Autodesk Inventor part; units mm, degrees
ref_plane "YZ Plane" through (0, 0, 0) normal (1, 0, 0) x (0, 1, 0)
ref_plane "XZ Plane" through (0, 0, 0) normal (0, 1, 0) x (-1, 0, 0)
ref_plane "XY Plane" through (0, 0, 0) normal (0, 0, 1) x (1, 0, 0)
sketch "Szkic1" plane through (0, 0, 0) normal (0, 1, 0) x (-1, 0, 0)
  line L0 (30, -20) -> (-30, -20)
  line L1 (-30, -20) -> (-30, 20)
  line L2 (-30, 20) -> (30, 20)
  line L3 (30, 20) -> (30, -20)
  line L4 (30, -20) -> (-30, 20) construction
  line L5 (-30, -20) -> (30, 20) construction
  point P0 (0, 0)
  dimension "d0" = 60
  dimension "d1" = 40
extrude "Wyciągnięcie proste1" add sketch "Szkic1" along normal blind 3
sketch "Szkic6" plane through (0, 3, 0) normal (0, 1, 0) x (1, 0, 0)
  line L0 (17.3578, -5.5734) -> (12.5578, -5.5734)
  line L1 (12.5578, -5.5734) -> (12.5578, 12.7266)
  line L2 (12.5578, 12.7266) -> (-10.1422, 12.7266)
  line L3 (-10.1422, -5.5734) -> (-10.1422, 12.7266)
  line L4 (-10.1422, -5.5734) -> (-14.9422, -5.5734)
  line L5 (-14.9422, -5.5734) -> (-14.9422, -8.2734)
  line L6 (-10.1422, -8.2734) -> (-14.9422, -8.2734)
  line L7 (-10.1422, -8.2734) -> (-10.1422, -10.0734)
  line L8 (-10.1422, -10.0734) -> (12.5578, -10.0734) construction
  line L9 (12.5578, -8.2734) -> (12.5578, -10.0734)
  line L10 (17.3578, -8.2734) -> (12.5578, -8.2734)
  line L11 (17.3578, -5.5734) -> (17.3578, -8.2734)
  line L12 (-8.8922, -2.4734) -> (11.3078, -2.4734)
  line L13 (-8.8922, 7.7266) -> (-8.8922, -2.4734)
  line L14 (11.3078, 7.7266) -> (-8.8922, 7.7266)
  line L15 (11.3078, -2.4734) -> (11.3078, 7.7266)
  line L16 (-30, -20) -> (30, -20)
  line L17 (30, -20) -> (30, 20)
  line L18 (30, -20) -> (30, 20)
  line L19 (-30, 20) -> (-30, -20)
  line L20 (-30, -20) -> (-14.5223, -20)
  line L21 (23.4752, -20) -> (30, -20)
  line L22 (-10.6422, 13.2266) -> (13.0578, 13.2266)
  line L23 (13.4777, 6.2814) -> (13.4777, -4.6535)
  line L24 (13.4777, -4.6535) -> (18.2777, -4.6535)
  line L25 (18.2777, -4.6535) -> (18.2777, -9.1933)
  line L26 (18.2777, -9.1933) -> (13.4777, -9.1933)
  line L27 (13.4777, -9.1933) -> (13.4777, -10.5734)
  line L28 (-10.6422, -10.5734) -> (-10.6422, -8.7734)
  line L29 (-10.6422, -8.7734) -> (-15.4422, -8.7734)
  line L30 (-15.4422, -8.7734) -> (-15.4422, -5.0734)
  line L31 (-15.4422, -5.0734) -> (-10.6422, -5.0734)
  line L32 (-10.6422, -5.0734) -> (-10.6422, 13.2266)
  line L33 (13.4777, -10.5734) -> (23.4752, -20)
  line L34 (-10.6422, -10.5734) -> (-14.5223, -20)
  line L35 (13.4777, 6.2814) -> (16.9504, 6.2814)
  line L36 (16.9504, 6.2814) -> (16.9504, 20)
  line L37 (13.0578, 13.2266) -> (13.0578, 20)
  line L38 (30, 20) -> (16.9504, 20)
  line L39 (13.0578, 20) -> (-30, 20)
  point P0 (0, 0)
  dimension "d4" = 0.5
extrude "Wyciągnięcie proste2" add sketch "Szkic6" along normal blind 13 contours L19 L39 L37 L22 L32 L31 L30 L29 L28 L34 L16 | L33 L27 L26 L25 L24 L23 L35 L36 L38 L17 L16
sketch "Szkic7" plane through (0, 3, 0) normal (0, 1, 0) x (1, 0, 0)
  line L0 (13.0578, 20) -> (13.0578, 13.2266)
  line L1 (13.0578, 13.2266) -> (-10.6422, 13.2266)
  line L2 (-10.6422, 13.2266) -> (-10.6422, -5.0734)
  line L3 (-10.6422, -5.0734) -> (-15.4422, -5.0734)
  line L4 (-15.4422, -5.0734) -> (-15.4422, -8.7734)
  line L5 (-15.4422, -8.7734) -> (-10.6422, -8.7734)
  line L6 (-10.6422, -8.7734) -> (-10.6422, -10.5734)
  line L7 (-10.6422, -10.5734) -> (-14.5223, -20)
  line L8 (-14.5223, -20) -> (23.4752, -20)
  line L9 (23.4752, -20) -> (13.4777, -10.5734)
  line L10 (13.4777, -10.5734) -> (13.4777, -9.1933)
  line L11 (13.4777, -9.1933) -> (18.2777, -9.1933)
  line L12 (18.2777, -9.1933) -> (18.2777, -4.6535)
  line L13 (18.2777, -4.6535) -> (13.4777, -4.6535)
  line L14 (13.4777, -4.6535) -> (13.4777, 6.2814)
  line L15 (13.4777, 6.2814) -> (16.9504, 6.2814)
  line L16 (16.9504, 6.2814) -> (16.9504, 20)
  line L17 (16.9504, 20) -> (13.0578, 20)
  line L18 (1.3504, -15.7734) -> (12.6578, -15.7734)
  line L19 (-12.7826, -15.7734) -> (18.9926, -15.7734)
  point P0 (0, 0)
  point P1 (12.6578, -15.7734)
  point P2 (1.3504, -15.7734)
extrude "Wyciągnięcie proste3" cut sketch "Szkic7" against normal blind 13 contours L19 L18 L9 L8 L7
sketch "Szkic8" plane through (0, 16, 0) normal (0, 1, 0) x (1, 0, 0)
  line L0 (-30, 20) -> (-30, -20)
  line L1 (-30, -20) -> (-14.5223, -20)
  line L2 (30, 20) -> (-30, 20)
  line L3 (-30, 0) -> (30, 0) construction
  line L4 (0, 20) -> (0, -29.6332) construction
  point P0 (0, 0)
  point P1 (-25, -15)
  point P2 (-25, 15)
  point P3 (25, 15)
  point P4 (25, -15)
  dimension "d9" = 5
  dimension "d10" = 5
hole "Otwór1" at (-25, 16, 15) at (-25, 16, -15) at (25, 16, -15) at (25, 16, 15) direction (0, -1, 0) diameter 4.134 depth 5 tip angle 118
sketch "Szkic9" plane through (0, 0, 0) normal (0, -1, 0) x (1, 0, 0)
  line L0 (30, 20) -> (30, -20)
  line L1 (30, -20) -> (-30, -20)
  line L2 (-30, -20) -> (-30, -17)
  line L3 (-30, -17) -> (30, -17)
  line L4 (30, -17) -> (30, -20)
  line L5 (18.9926, 15.7734) -> (-12.7826, 15.7734)
  line L6 (30, 20) -> (23.4752, 20)
  line L7 (23.4752, 17) -> (30, 17)
  line L8 (30, 17) -> (30, 20)
  line L9 (23.4752, 20) -> (18.9926, 15.7734)
  line L10 (23.4752, 20) -> (23.4752, 17)
  line L11 (-30, 20) -> (-14.5223, 20)
  line L12 (-30, 20) -> (-14.5223, 20)
  line L13 (-14.5223, 17) -> (-30, 17)
  line L14 (-30, 17) -> (-30, 20)
  line L15 (-14.5223, 20) -> (-10.6422, 10.5734)
  line L16 (-14.5223, 20) -> (-14.5223, 17)
  point P0 (0, 0)
  dimension "d18" = 60
  dimension "d19" = 3
  dimension "d31" = 3
  dimension "d32" = 3
extrude "Wyciągnięcie proste4" add sketch "Szkic9" along normal blind 3
sketch "Szkic10" plane through (0, 16, 0) normal (0, 1, 0) x (1, 0, 0)
  line L0 (-30, 20) -> (-30, -20)
  line L1 (30, -20) -> (30, 20)
  point P0 (0, 0)
  point P1 (-20, 0)
  point P2 (20, 0)
  dimension "d22" = 10
  dimension "d23" = 10
hole "Otwór2" at (-20, 16, 0) at (20, 16, 0) direction (0, -1, 0) diameter 4.134 end through all
properties part number "Podstawa"
The model under review builds one solid part; all positions refer to its coordinate system, in mm. A direction names the side the tool comes from. Round coordinates to 2 decimals unless told otherwise and drop trailing zeros. Loops run counter-clockwise (first coordinate to the right, second up) from the corner with the lowest first, then second, coordinate; pieces in that order, holes last.
Item 1: Clearance check with flat-ended pins moving along their axes: pin 1 Ø12 at (x, z) = (9.5, -4.5) entering from +Y; pin 2 Ø1.4 at (x, y) = (-12, 12) entering from +Z; pin 3 Ø5 at (x, y) = (10.5, 4) entering from +Z; pin 4 Ø6 at (x, z) = (-13, -10.5) entering from -Y. State where each tip first meets the part, or that it passes through.
Determined:
pin 1: stops at y = 16
pin 2: stops at z = 15.57
pin 3: stops at z = 15.77
pin 4: stops at y = 0
Item 2: For faces 4 (the face through (-26.743, 13.465, 16.111)), 5 (the face through (13.478, 9, -1)), 6 (the face through (1, 9, -13.227)), 7 (the face through (23.475, -1, 19)), list the 3-axis set-ups (+Z, -Z, +X, -X, +Y, -Y) from which the entire face can be reached by the end or side of a thin tool; tool diameter is ignored.
Determined:
face 4: +Y
face 5: +Z, -Z, +Y
face 6: +Z, +Y
face 7: +Z, -Y
Item 3: Take a section at A-A (y = 9). Write out the cut boundary in (x, z).
Determined:
outline: (-30, -20) - (13.06, -20) - (13.06, -13.23) - (-10.64, -13.23) - (-10.64, 5.07) - (-15.44, 5.07) - (-15.44, 8.77) - (-10.64, 8.77) - (-10.64, 10.57) - (-14.52, 20) - (-30, 20) - close; (13.48, -6.28) - (16.95, -6.28) - (16.95, -20) - (30, -20) - (30, 20) - (23.48, 20) - (13.48, 10.57) - (13.48, 9.19) - (18.28, 9.19) - (18.28, 4.65) - (13.48, 4.65) - close; hole circle Ø4.13 at (-20, 0); hole circle Ø4.13 at (20, 0)
Item 4: Take a section at D-D (x = 20). Write out the cut boundary in (y, z), then the cut area to 3 significant figures.
Determined:
outline: (-3, -20) - (16, -20) - (16, -2.07) - (0, -2.07) - (0, -17) - (-3, -17) - close; (0, 2.07) - (16, 2.07) - (16, 16.72) - (0, 16.72) - close
area: 530 mm2
Item 5: Take a section at C-C (y = 14). Write out the cut boundary in (x, z), then the cut area to 3 significant figures.
Determined:
outline: (-30, -20) - (13.06, -20) - (13.06, -13.23) - (-10.64, -13.23) - (-10.64, 5.07) - (-15.44, 5.07) - (-15.44, 8.77) - (-10.64, 8.77) - (-10.64, 10.57) - (-14.52, 20) - (-30, 20) - close; (13.48, -6.28) - (16.95, -6.28) - (16.95, -20) - (30, -20) - (30, 20) - (23.48, 20) - (13.48, 10.57) - (13.48, 9.19) - (18.28, 9.19) - (18.28, 4.65) - (13.48, 4.65) - close; hole circle Ø4.13 at (-25, -15); hole circle Ø4.13 at (-25, 15); hole circle Ø4.13 at (-20, 0); hole circle Ø4.13 at (20, 0); hole circle Ø4.13 at (25, -15); hole circle Ø4.13 at (25, 15)
area: 1,360 mm2
Item 6: Take a section at B-B (z = 0). Write out the cut boundary in (x, y), then the cut area to 3 significant figures.
Determined:
outline: (-30, 0) - (-22.07, 0) - (-22.07, 16) - (-30, 16) - close; (-17.93, 0) - (17.93, 0) - (17.93, 16) - (13.48, 16) - (13.48, 3) - (-10.64, 3) - (-10.64, 16) - (-17.93, 16) - close; (22.07, 0) - (30, 0) - (30, 16) - (22.07, 16) - close
area: 514 mm2
Item 7: For line 1 (Z direction, x = 25, y = 13.6); line 2 (X direction, y = 12.25, z = 0); line 3 (X direction, y = 13.45, z = -15), list the stretches that pass through material, from the lowest coordinate up.
Determined:
line 1: z = -20 to -17.07, -12.93 to 12.93, 17.07 to 20
line 2: x = -30 to -22.07, -17.93 to -10.64, 13.48 to 17.93, 22.07 to 30
line 3: x = -30 to -27.07, -22.93 to 13.06, 16.95 to 22.93, 27.07 to 30
Item 8: Mouldability with a two-part tool opening along Z and no side actions: class faces 1 (the face through (-22, -3, 19)), 2 (the face through (23.257, 13.465, 16.111)), 3 (the face through (15, 9, -6.281)) as released by +Z, released by -Z, zero draft, split by the parting line, or undercut.
Determined:
face 1: zero draft
face 2: undercut
face 3: released by -Z
